Source: three-view drawing plus pictorial views. Frame: mm from the lowest corner of the part. A direction names the side the tool comes from. Coordinates: 2 decimals unless noted, no trailing zeros. Write each loop counter-clockwise with the first axis right and the second up, starting at its lowest first coordinate (ties: lowest second). Pieces come first, ordered by that corner, then holes. Notation, with made-up numbers: M -27,10.25 L -6,10.25 A12 cw -6,15.25 Z; hole C 24,50.5 d1. An arc over 180 degrees is marked long. Answer as a JSON object with one key per item and string values. Group by question number.
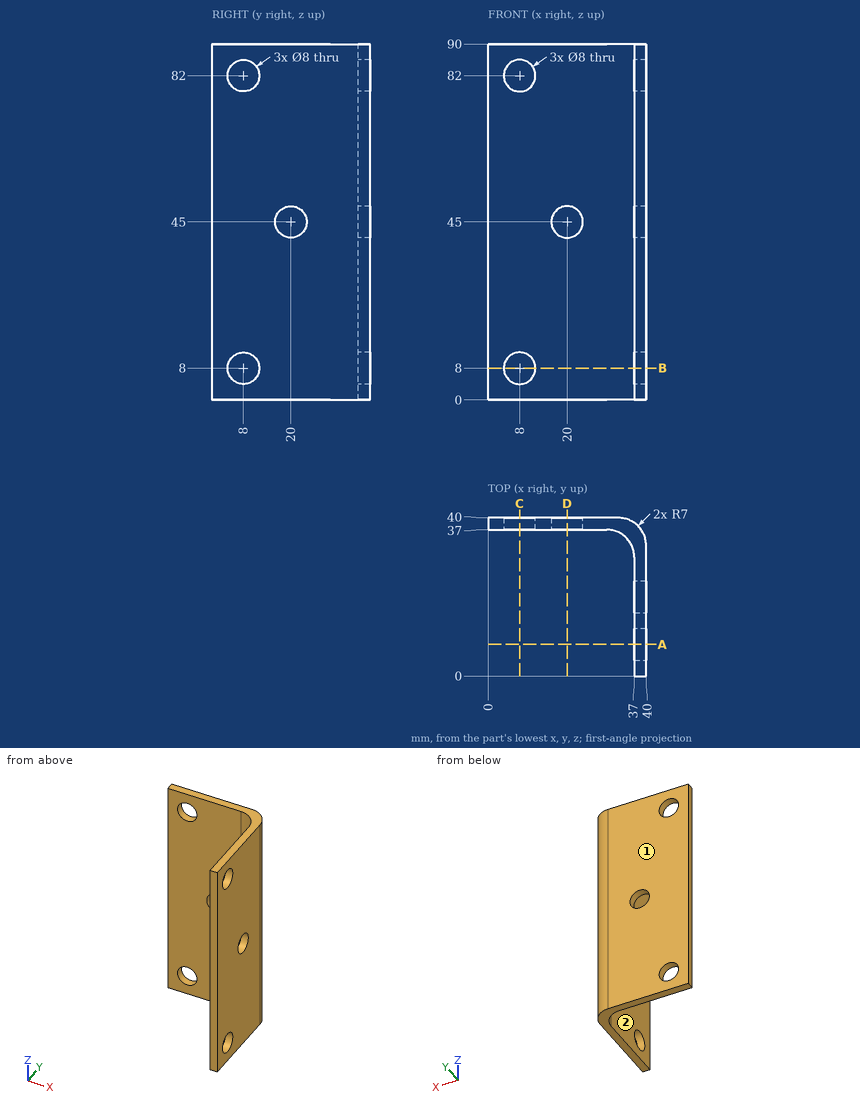
Q1. Section D-D, the plane x = 20. Return the cut outline in (y, z).
Q2. Section B-B, the plane z = 8. Return the cut outline in (x, y).
Q3. Section A-A, the plane y = 8. Return the cut outline in (x, z), and give its area (3 significant figures).
Q4. Pin query (flat end, axial travel): pin 1 Ø6.5 at (x, z) = (20, 45) entering from +Y; pin 2 Ø13 at (y, z) = (8, 8) entering from -X; pin 3 Ø10.5 at (x, z) = (8, 8) entering from -Y. Return the tip coordinate at first contact, or that it passes through.
Q5. Access query for the marked faces 1 and 2. Directions: +Z, -Z, +X, -X, +Y, -Y. A direction counts if a zero-diameter tool reaches every point of the face in a straight line with its end or side. Return the directions, or none.
Q6. Line query: line 1 (Z direction, x = 20, y = 39.35); line 2 (Y direction, x = 6, z = 28). Output: solid intervals per line, ascending. Write a range as from..to.
Filled in:
{
 "1": {"outline": "M 37,0 L 40,0 L 40,41 L 37,41 Z; M 37,49 L 40,49 L 40,90 L 37,90 Z"},
 "2": {"outline": "M 0,37 L 4,37 L 4,40 L 0,40 Z; M 12,37 L 30,37 A7 cw 37,30 L 37,12 L 40,12 L 40,33 A7 ccw 33,40 L 12,40 Z; M 37,0 L 40,0 L 40,4 L 37,4 Z"},
 "3": {"outline": "M 37,0 L 40,0 L 40,4 L 37,4 Z; M 37,12 L 40,12 L 40,78 L 37,78 Z; M 37,86 L 40,86 L 40,90 L 37,90 Z", "area": "222 mm^2"},
 "4": {"pin 1": "through", "pin 2": "x = 37", "pin 3": "y = 37"},
 "5": {"face 1": "+Z, -Z, +X, -X, +Y", "face 2": "+Z, -Z, -X, -Y"},
 "6": {"line 1": "0..41, 49..90", "line 2": "37..40"}
}
